```python
from build123d import *

# Parameters (mm, degrees)
SKETCH1_R           = 15.875
SKETCH1_R_2         = 7.5
SKETCH1_W           = 55
SKETCH1_H           = 3.175
BOSS_EXTRUDE1_DEPTH = 3.175


with BuildPart() as part:
    # Sketch1 → Boss-Extrude1 (new body)
    with BuildSketch(Plane.XY):
        with BuildLine():
            Line((13.470384182, 13.470384182), (267.470384182, 13.470384182))
            ThreePointArc((267.470384182, 13.470384182), (280.940768363, 0), (267.470384182, -13.470384182))
            Line((267.470384182, -13.470384182), (13.470384182, -13.470384182))
            ThreePointArc((13.470384182, -13.470384182), (-19.05, 0), (13.470384182, 13.470384182))
        make_face()
        Circle(SKETCH1_R, mode=Mode.SUBTRACT)
        with Locations((267.470384182, 0)):
            Circle(SKETCH1_R_2, mode=Mode.SUBTRACT)
        with Locations((191.720384182, 0)):
            Circle(SKETCH1_R_2, mode=Mode.SUBTRACT)
        Polygon((122.588897068, 0), (118.001577828, -11.0885753), (120.001577828, -11.0885753), (129.176216309, 11.0885753), (127.176216309, 11.0885753), align=None, mode=Mode.SUBTRACT)
        with Locations((80.970384182, 0)):
            Rectangle(SKETCH1_W, SKETCH1_H, mode=Mode.SUBTRACT)
        Polygon((134.176216309, 11.0885753), (125.001577828, -11.0885753), (123.001577828, -11.0885753), (127.588897068, 0), (132.176216309, 11.0885753), align=None, mode=Mode.SUBTRACT)
        Polygon((139.176216309, 11.0885753), (130.001577828, -11.0885753), (128.001577828, -11.0885753), (132.588897068, 0), (137.176216309, 11.0885753), align=None, mode=Mode.SUBTRACT)
        Polygon((144.176216309, 11.0885753), (135.001577828, -11.0885753), (133.001577828, -11.0885753), (137.588897068, 0), (142.176216309, 11.0885753), align=None, mode=Mode.SUBTRACT)
        Polygon((149.176216309, 11.0885753), (140.001577828, -11.0885753), (138.001577828, -11.0885753), (142.588897068, 0), (147.176216309, 11.0885753), align=None, mode=Mode.SUBTRACT)
        Polygon((154.176216309, 11.0885753), (145.001577828, -11.0885753), (143.001577828, -11.0885753), (147.588897068, 0), (152.176216309, 11.0885753), align=None, mode=Mode.SUBTRACT)
        Polygon((159.176216309, 11.0885753), (150.001577828, -11.0885753), (148.001577828, -11.0885753), (152.588897068, 0), (157.176216309, 11.0885753), align=None, mode=Mode.SUBTRACT)
        Polygon((164.176216309, 11.0885753), (155.001577828, -11.0885753), (153.001577828, -11.0885753), (157.588897068, 0), (162.176216309, 11.0885753), align=None, mode=Mode.SUBTRACT)
        Polygon((169.176216309, 11.0885753), (160.001577828, -11.0885753), (158.001577828, -11.0885753), (162.588897068, 0), (167.176216309, 11.0885753), align=None, mode=Mode.SUBTRACT)
        Polygon((174.176216309, 11.0885753), (165.001577828, -11.0885753), (163.001577828, -11.0885753), (167.588897068, 0), (172.176216309, 11.0885753), align=None, mode=Mode.SUBTRACT)
    extrude(amount=BOSS_EXTRUDE1_DEPTH)


solid = part.part
```
Geometry check sheet. Reference: the model listing, model coordinates, mm. A direction names the side the tool comes from. Coordinates: 2 decimals unless noted, no trailing zeros. Write each loop counter-clockwise with the first axis right and the second up, starting at its lowest first coordinate (ties: lowest second). Pieces come first, ordered by that corner, then holes. Notation, with made-up numbers: M 15.5,41 L 32.5,41 A25 cw 32.5,67 Z; hole C 44,26.25 d2. An arc over 180 degrees is marked long. One line per item, written item: value. Start each with the question number.
(1) Sectioned sample at B-B, the plane z = 2.65. State how many separate pieces and enclosed holes the cut face has, and give its area (3 significant figures).
(2) Release check for a two-part mould opening along Y. For faces 1 (the face through (139.653, 0.155, 1.565)), 2 (the face through (133, 5, 0)), 3 (the face through (280.938, 0.296, 1.565)) record: released by +Y, released by -Y, zero draft, split by the parting line, or undercut.
(3) Scan lines: line 1 along Y through (x, z) = (0, 2.4) (3 decimals); line 2 along Y through (x, z) = (191.5, 1.7); line 3 along Y through (x, z) = (150, 2.1). Record each from-to range of solid material in increasing order. Write a range as [from, to].
(4) Sectioned sample at A-A, the plane x = 0. Enter the section's corners in (y, z) (3 decimals), and give its area (3 significant figures).
(5) Depth check by flat-ended pin: pin 1 (1.6 mm diameter, centred on x = 71, z = 1.5, fed in from -Y); pin 2 (1.6 mm diameter, centred on x = 129, z = 1.5, fed in from +Y); pin 3 (1 mm diameter, centred on y = -0.5, z = 2, fed in from -X). Enter the tip coordinate at first touch or a pass-through.
(6) Tool access check on faces 4 (the face through (133, 5, 3.175)), 5 (the face through (169.653, 0.155, 1.565)). Record the directions out of +Z, -Z, +X, -X, +Y, -Y that give a thin tool (end or side, any length) a straight path to the whole face; none if there is none.
Filled sheet:
1. separate pieces: 1
1. enclosed holes: 14
1. area: 6,400 mm²
2. face 1: undercut
2. face 2: zero draft
2. face 3: split by the parting line
3. line 1: [-19.05, -15.875], [15.875, 19.05]
3. line 2: [-13.47, -7.5], [7.5, 13.47]
3. line 3: [-13.47, -11.09], [-6.26, 0.99], [5.83, 13.47]
4. outline: M -19.05,0 L -15.875,0 L -15.875,3.175 L -19.05,3.175 Z; M 15.875,0 L 19.05,0 L 19.05,3.175 L 15.875,3.175 Z
4. area: 20.2 mm²
5. pin 1: y = -13.47
5. pin 2: y = 13.47
5. pin 3: x = -19.05
6. face 4: +Z, +X, -X, +Y, -Y
6. face 5: +Z, -Z
